Verification items for the finished model (mm, model axes). A direction names the side the tool comes from. Give positions to 0.01 mm unless a question says otherwise; leave off trailing zeros. Loops run counter-clockwise (first coordinate to the right, second up) from the corner with the lowest first, then second, coordinate; pieces in that order, holes last. Notation, with made-up numbers: M 69,23.5 L 85,23.5 A27 ccw 85,39.5 Z; hole C -21,-10.5 d6. An arc over 180 degrees is marked long. Put each result on its own line as item: value. Start each with the question number.
from build123d import *

# Parameters (mm, degrees)
F0_W     = 43.043024838
F0_H     = 43.7836721539
F1_DEPTH = 800
F2_DEPTH = 200
F3_DEPTH = 600
F4_T     = -18


with BuildPart() as f1:
    # F0 (on Top) → F1 (new body)
    with BuildSketch(Plane.XY):
        with Locations((21.521512419, -21.891836077)):
            Rectangle(F0_W, F0_H)
    extrude(amount=F1_DEPTH)

    # F2 (add): a face of the model
    f2_faces = [f1.faces().sort_by_distance(p)[0] for p in [
        (0, -21.891836077, 400),
    ]]
    extrude(f2_faces, amount=-F2_DEPTH)

    # F3 (add): a face of the model
    f3_faces = [f1.faces().sort_by_distance(p)[0] for p in [
        (100, -43.7836721539, 400),
    ]]
    extrude(f3_faces, amount=-F3_DEPTH)

    # F4
    f4_openings = [f1.faces().sort_by_distance(p)[0] for p in [
        (100, -43.783672, 400),
    ]]
    offset(amount=F4_T, openings=f4_openings)


solid = f1.part
Q1. Cross-section at B-B, the plane z = 426. Record the boundary of the cut face in (x, y), then the cut area to 3 significant figures.
Q2. Scan lines: L1, parallel to X at y = 167.5, z = 142; L2, parallel to Z at x = 114.5, y = 311.5; L3, parallel to Y at x = 138.5, z = 384.5. Record each from-to range of solid material in increasing order.
Q3. Set-up check for faces 1 (the face through (200, 252, 394)), 2 (the face through (99, 251, 782)): record each of +Z, -Z, +X, -X, +Y, -Y from which the full face is reachable in a straight line by a thin tool's end or side.
Q4. Go/stop test with a flat-tipped pin: pin 1 (5 mm diameter, centred on x = 123.5, z = 268, fed in from -Y). Record where the tip stops, or that it passes through.
Q5. Cross-section at C-C, the plane x = 60.5. Record the boundary of the cut face in (y, z), then the cut area to 3 significant figures.
Q6. Cross-section at A-A, the plane y = 188. Record the boundary of the cut face in (x, z), then the cut area to 3 significant figures.
Q7. Release check for a two-part mould opening along X. For faces 3 (the face through (0, 252, 394)), 4 (the face through (99, 251, 18)), 5 (the face through (99, 260, 800)) record: pulls with the +X half, pulls with the -X half, needs draft (parallel to the pull), parting line crosses it, or undercut.
Ans:
1. outline: M 0,-43.78 L 18,-43.78 L 18,538.22 L 182,538.22 L 182,-43.78 L 200,-43.78 L 200,556.22 L 0,556.22 Z
1. area: 24,600 mm^2
2. L1: x = 0 to 18, 182 to 200
2. L2: z = 0 to 18, 782 to 800
2. L3: y = 538.22 to 556.22
3. face 1: +Z, -Z, +X, +Y, -Y
3. face 2: -Y
4. pin 1: stops at y = 538.22
5. outline: M -43.78,0 L 556.22,0 L 556.22,800 L -43.78,800 L -43.78,782 L 538.22,782 L 538.22,18 L -43.78,18 Z
5. area: 35,400 mm^2
6. outline: M 0,0 L 200,0 L 200,800 L 0,800 Z; hole M 18,18 L 182,18 L 182,782 L 18,782 Z
6. area: 34,700 mm^2
7. face 3: pulls with the -X half
7. face 4: undercut
7. face 5: needs draft
